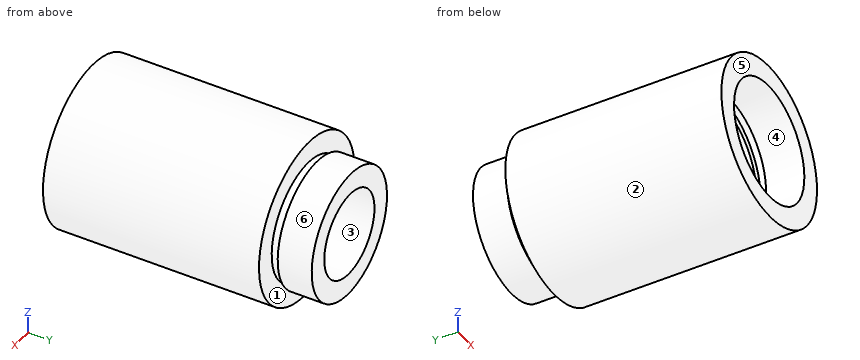
from build123d import *


with BuildPart() as part:
    # 草图1 → 旋转1 (revolve)
    with BuildSketch(Plane.XY, mode=Mode.PRIVATE) as revolve_1_sk:
        Polygon((7, 26.4), (7.5, 26.4), (7.5, 30.4), (5, 30.4), (5, 23.4), (6.85, 23.4), (6.85, 22.4), (6.75, 22.4), (6.75, 5.5), (7.6, 5.5), (7.6, 4.5), (7, 4.5), (7, 0), (9.525, 0), (9.525, 25.4), (7, 25.4), align=None)
    revolve(revolve_1_sk.sketch.rotate(Axis((0, 161.376166943, 0), (0, -1, 0)), 90), axis=Axis((0, 161.376166943, 0), (0, -1, 0)))  # turned: the seam where the file's is


solid = part.part
Verification items for the finished model (mm, model axes). Face numbers are marked on the shaded views. A direction names the side the tool comes from. Coordinates: 2 decimals unless noted, no trailing zeros. Order: outer loops, then holes, each group sorted by start corner. A loop starts at its lowest first (then second) coordinate and runs counter-clockwise, first axis right, second up.
Item 1: Access from +Z, -Z, +X, -X, +Y, -Y to the whole of each face (thin tool, end or side, straight path). Record for the marked faces 5 and 6.
Filled in:
face 5: +Z, -Z, +X, -X, -Y
face 6: +Y
Item 2: Section check C-C, the plane y = 8. Enter the section's corners in (x, z) (3 decimals), then the cut area to 3 significant figures.
Filled in:
outline: circle Ø19.05 at (0, 0); hole circle Ø13.5 at (0, 0)
area: 142 mm2
Item 3: Material ranges on L1, parallel to X at y = 27.5, z = 0; L2, parallel to Y at x = -7, z = -1.5; L3, parallel to X at y = 25, z = 0 (3 decimals), recorded low to high.
Filled in:
L1: x = -7.5 to -5, 5 to 7.5
L2: y = 0 to 4.5, 5.5 to 25.4, 26.4 to 30.4
L3: x = -9.525 to -5, 5 to 9.525
Item 4: Depth check by flat-ended pin: pin 1 (5 mm diameter, centred on x = 7.5, y = 23.5, fed in from -Z); pin 2 (4.5 mm diameter, centred on x = 1, z = -2.5, fed in from -Y); pin 3 (2 mm diameter, centred on y = 19, z = -2.5, fed in from +X); pin 4 (7.5 mm diameter, centred on x = -3, z = 0.5, fed in from -Y). Enter the tip coordinate at first touch or a pass-through.
Filled in:
pin 1: stops at z = -8.11
pin 2: passes through
pin 3: stops at x = 9.41
pin 4: stops at y = 5.5
Item 5: Release check for a two-part mould opening along Z. For the marked faces 1, 2, 3 and 4 record: +Z half, -Z half, draft (parallel to the pull), parting line (faces both ways), or undercut.
Filled in:
face 1: draft
face 2: parting line
face 3: undercut
face 4: undercut
Item 6: Section check D-D, the plane z = -5.5. Enter the section's corners in (x, y) (3 decimals).
Filled in:
outline: (-7.777, 0) - (-4.33, 0) - (-4.33, 4.5) - (-5.245, 4.5) - (-5.245, 5.5) - (-3.913, 5.5) - (-3.913, 22.4) - (-4.083, 22.4) - (-4.083, 23.4) - (4.083, 23.4) - (4.083, 22.4) - (3.913, 22.4) - (3.913, 5.5) - (5.245, 5.5) - (5.245, 4.5) - (4.33, 4.5) - (4.33, 0) - (7.777, 0) - (7.777, 25.4) - (4.33, 25.4) - (4.33, 26.4) - (5.099, 26.4) - (5.099, 30.4) - (-5.099, 30.4) - (-5.099, 26.4) - (-4.33, 26.4) - (-4.33, 25.4) - (-7.777, 25.4) - close
